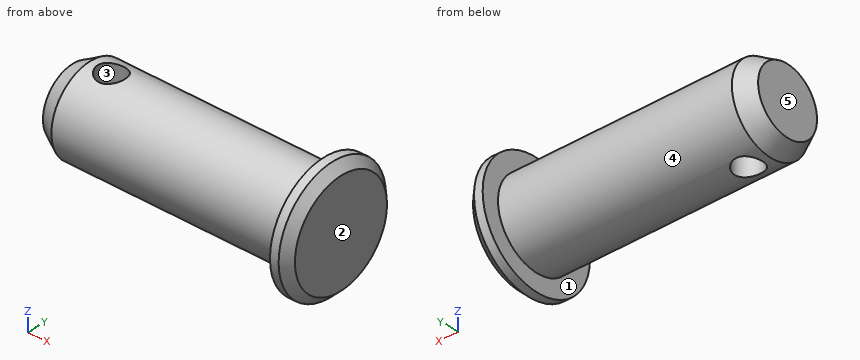
from build123d import *

# Parameters (mm, degrees)
SKETCH1_W              = 29
SKETCH1_H              = 5
HEAD_CHAMFER_SIZE      = 2
HEAD_CHAMFER_SIZE2     = 1.154700538
SKETCH21_R             = 1.6
R_CLIP_HOLE_DEPTH      = 8
R_CLIP_HOLE_DEPTH_BACK = 8


with BuildPart() as part:
    # Sketch1 → Body Revolve (revolve)
    with BuildSketch(Plane.XY):
        with Locations((-14.5, 2.5)):
            Rectangle(SKETCH1_W, SKETCH1_H)
    revolve(axis=Axis((0, 0, 0), (-1, 0, 0)))

    # Sketch14 → Head Revolve (revolve)
    with BuildSketch(Plane.XY):
        Polygon((0, 0), (2, 0), (2, 6), (1, 7), (0, 7), align=None)
    revolve(axis=Axis((0, 0, 0), (1, 0, 0)))

    # Head Chamfer
    head_chamfer_edges = [part.edges().sort_by_distance(p)[0] for p in [
        (-29, -5, 0),
    ]]
    head_chamfer_side = [part.faces().sort_by_distance(p)[0] for p in [
        (-14.5, -5, 0),
    ]]
    chamfer(head_chamfer_edges, length=HEAD_CHAMFER_SIZE, length2=HEAD_CHAMFER_SIZE2, reference=head_chamfer_side[0])

    # Sketch21 → R Clip Hole (cut, two sides)
    with BuildSketch(Plane.XY) as r_clip_hole_sk:
        with Locations((-24.5, 0)):
            Circle(SKETCH21_R)
    extrude(amount=R_CLIP_HOLE_DEPTH, mode=Mode.SUBTRACT)
    extrude(r_clip_hole_sk.sketch, amount=-R_CLIP_HOLE_DEPTH_BACK, mode=Mode.SUBTRACT)


solid = part.part
Source: CAD feature listing. Evaluate the final solid. Frame: model axes, mm. Face numbers are marked on the shaded views. A direction names the side the tool comes from. Give positions to 0.01 mm unless a question says otherwise; leave off trailing zeros. Write each loop counter-clockwise with the first axis right and the second up, starting at its lowest first coordinate (ties: lowest second). Pieces come first, ordered by that corner, then holes. Notation, with made-up numbers: M -2,70 L 3,70 A25 cw 3,103 Z; hole C -36.75,33.5 d4. An arc over 180 degrees is marked long. Return JSON: item names as keys, results as strings. Group by question number.
1) Cut plane C-C, the plane x = -17. Output: boundary loops of the cut face in (y, z), plus the area to 3 significant figures.
2) Pin query (flat end, axial travel): P1, Ø5, axis at x = -24.5, y = 0, coming from the -Z side; P2, Ø2, axis at x = -20.5, z = -4.5, coming from the +Y side; P3, Ø4, axis at x = -10.5, z = -1, coming from the -Y side. Return the tip coordinate at first contact, or that it passes through.
3) Cut plane D-D, the plane x = -24.5. Output: boundary loops of the cut face in (y, z), plus the area to 3 significant figures.
4) Set-up query: the marked faces 4 and 5. Return all of +Z, -Z, +X, -X, +Y, -Y with unobstructed straight access to the full face (end or side cutting, diameter ignored); none if empty.
5) Cut plane B-B, the plane z = 0. Output: boundary loops of the cut face in (x, y), plus the area to 3 significant figures.
6) Cut plane A-A, the plane y = 0. Output: boundary loops of the cut face in (x, z), plus the area to 3 significant figures.
7) Material intervals for line 1 along X through (y, z) = (0, 1.5); line 2 along Y through (x, z) = (-22.5, 0.25); line 3 along X through (y, z) = (-0.5, 2), sorted ascending. Write a range as [from, to].
8) Pull-direction query (X, two-part tool) for the marked faces 1, 2 and 3; classes: pulls with the +X half, pulls with the -X half, needs draft (parallel to the pull), parting line crosses it, or undercut.
Recorded:
{
 "1": {"outline": "C 0,0 d10", "area": "78.5 mm²"},
 "2": {"P1": "stops at z = -5", "P2": "stops at y = 3.57", "P3": "stops at y = -5"},
 "3": {"outline": "M -1.6,-4.74 L -1.6,4.74 A5 ccw Z; M 1.6,-4.74 A5 ccw 1.6,4.74 Z", "area": "47.1 mm²"},
 "4": {"face 4": "-X", "face 5": "+Z, -Z, -X, +Y, -Y"},
 "5": {"outline": "M -29,-3.85 L -27,-5 L 0,-5 L 0,-7 L 1,-7 L 2,-6 L 2,6 L 1,7 L 0,7 L 0,5 L -27,5 L -29,3.85 Z; hole C -24.5,0 d3.2", "area": "307 mm²"},
 "6": {"outline": "M -29,-3.85 L -27,-5 L -26.1,-5 L -26.1,5 L -27,5 L -29,3.85 Z; M -22.9,-5 L 0,-5 L 0,-7 L 1,-7 L 2,-6 L 2,6 L 1,7 L 0,7 L 0,5 L -22.9,5 Z", "area": "283 mm²"},
 "7": {"line 1": "x = [-29, -26.1], [-22.9, 2]", "line 2": "y = [-4.99, 4.99]", "line 3": "x = [-29, -26.02], [-22.98, 2]"},
 "8": {"face 1": "pulls with the -X half", "face 2": "pulls with the +X half", "face 3": "undercut"}
}
